Study the drawing (mm; zero at the part's minimum x, y, z) and answer. A direction names the side the tool comes from. Round coordinates to 2 decimals unless told otherwise and drop trailing zeros. Write each loop counter-clockwise with the first axis right and the second up, starting at its lowest first coordinate (ties: lowest second). Pieces come first, ordered by that corner, then holes. Notation, with made-up numbers: (-8, 61) - (41, 61) arc R16 ccw to (41, 66) - close; hole circle Ø2 at (54.5, -36). An arc over 180 degrees is marked (long way). Return JSON: item names as keys, results as strings. Group by question number.
(1) Section D-D, the plane x = 21.59 is taken. Write down the section's boundary in (y, z), then the cut area to 3 significant figures.
(2) Which of the six approach directions +Z, -Z, +X, -X, +Y, -Y give full straight-line access (tool end or side, diameter ignored) to the marked faces 1 and 2?
(3) Section A-A, the plane x = 6.35 is taken. Write down the section's boundary in (y, z) (3 decimals).
(4) Section B-B, the plane z = 6.35 is taken. Write down the section's boundary in (x, y) (3 decimals).
(5) Determine the mould class of the marked faces 3, 4 and 5 for opening direction X: +X half, -X half, draft (parallel to the pull), parting line (faces both ways), or undercut.
(6) Find the intervals of material crossed by line 1 along Z through (x, y) = (6.35, 2.1) (3 decimals); line 2 along X through (y, z) = (2, 7.25); line 3 along Y through (x, z) = (33.5, 3.5), in increasing order. Write a range as [from, to].
(7) Section C-C, the plane z = 2.25 is taken. Write down the section's boundary in (x, y), then the cut area to 3 significant figures.
(8) Each of these flat-tipped pins is pushed along its axis until it touches: pin 1 (4 mm diameter, centred on x = 24, z = 11, fed in from +Y); pin 2 (6.5 mm diameter, centred on x = 35, z = 5, fed in from +Y); pin 3 (1 mm diameter, centred on x = 27.5, z = 10.5, fed in from +Y); pin 4 (2 mm diameter, centred on x = 31, y = 8, fed in from -Z). Where does it stop, or does it pass through?
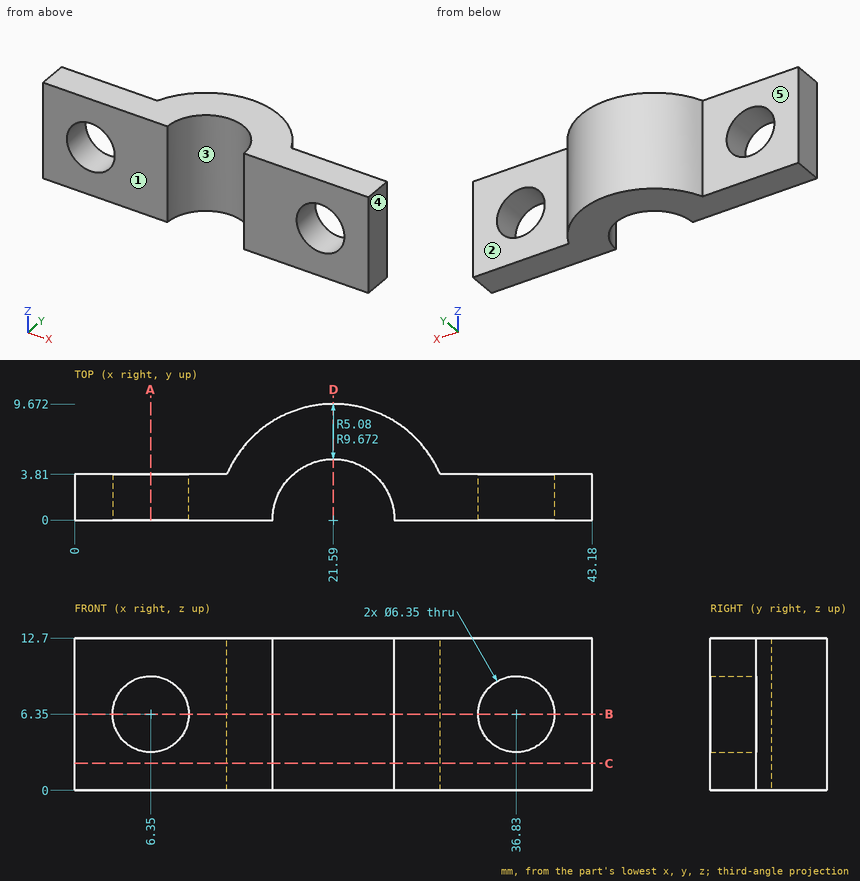
Working result:
{
 "1": {"outline": "(5.08, 0) - (9.67, 0) - (9.67, 12.7) - (5.08, 12.7) - close", "area": "58.3 mm^2"},
 "2": {"face 1": "+Z, -Z, +X, -X, -Y", "face 2": "+Z, -Z, +X, +Y"},
 "3": {"outline": "(0, 0) - (3.81, 0) - (3.81, 3.175) - (0, 3.175) - close; (0, 9.525) - (3.81, 9.525) - (3.81, 12.7) - (0, 12.7) - close"},
 "4": {"outline": "(0, 0) - (3.175, 0) - (3.175, 3.81) - (0, 3.81) - close; (9.525, 0) - (16.51, 0) arc R5.08 cw to (26.67, 0) - (33.655, 0) - (33.655, 3.81) - (30.48, 3.81) arc R9.672 ccw to (12.7, 3.81) - (9.525, 3.81) - close; (40.005, 0) - (43.18, 0) - (43.18, 3.81) - (40.005, 3.81) - close"},
 "5": {"face 3": "undercut", "face 4": "+X half", "face 5": "draft"},
 "6": {"line 1": "z = [0, 3.175], [9.525, 12.7]", "line 2": "x = [0, 3.31], [9.39, 16.92], [26.26, 33.79], [39.87, 43.18]", "line 3": "y = [0, 3.81]"},
 "7": {"outline": "(0, 0) - (16.51, 0) arc R5.08 cw to (26.67, 0) - (43.18, 0) - (43.18, 3.81) - (30.48, 3.81) arc R9.67 ccw to (12.7, 3.81) - (0, 3.81) - close", "area": "199 mm^2"},
 "8": {"pin 1": "stops at y = 9.66", "pin 2": "stops at y = 3.81", "pin 3": "stops at y = 8.02", "pin 4": "passes through"}
}
